Build history of the part. All positions in model axes, mm. A direction names the side the tool comes from. Round coordinates to 2 decimals unless told otherwise and drop trailing zeros. Write each loop counter-clockwise with the first axis right and the second up, starting at its lowest first coordinate (ties: lowest second). Pieces come first, ordered by that corner, then holes. Notation, with made-up numbers: M 23.25,38 L 72.25,38 A13 cw 72.25,61 Z; hole C 8.5,16 d2. An arc over 180 degrees is marked long. Use a Markdown table: item, result.
from build123d import *

# Parameters (mm, degrees)
F2_DEPTH    = 12.5
F3_T1_DEPTH = 46.550163213
F3_T3_DEPTH = 50.7168298797
F4_R        = 1
F4_R_2      = 0.99999


# Not quite as in the source:
# - a fillet or chamfer that OpenCascade refuses, or shapes differently, is made with other operations: its cross-section is extruded or revolved along the edge and cut away or added
# - a fillet or chamfer is up to 0.001 mm smaller than in the source, because OpenCascade refuses the exact size


with BuildPart() as f2:
    # F1 (on Front) → F2 (new body, symmetric)
    with BuildSketch(Plane.XZ):
        Polygon((0, 2), (0, 0), (20.8333333333, 0), (20.8333333333, 8), (18.3333333333, 8), (18.3333333333, 6), (15, 6), (15, 4), (10, 4), (10, 2), align=None)
    extrude(amount=F2_DEPTH, both=True)

    # F3: chamfer of 5 on 4 edges, made by hand

    # F3_s2 → F3_t1 (cut)
    with BuildSketch(Plane.YZ.offset(-12.8584149398)):
        Polygon((-12.5, 5), (-7.5, 0), (-12.5, 0), align=None)
        Polygon((7.5, 0), (12.5, 5), (12.5, 0), align=None)
    extrude(amount=F3_T1_DEPTH, mode=Mode.SUBTRACT)

    # F3_s4 → F3_t3 (cut)
    with BuildSketch(Plane.XZ.offset(-25.3584149398)):
        Polygon((0, 5), (5, 0), (0, 0), align=None)
        Polygon((20.8333333333, 5), (15.8333333333, 0), (20.8333333333, 0), align=None)
    extrude(amount=F3_T3_DEPTH, mode=Mode.SUBTRACT)

    # F4 (call 1 of 10: OpenCascade refuses the feature's edges together)
    f4_edges = [f2.edges().sort_by_distance(p)[0] for p in [
        (6.5, -9.5, 2),
    ]]
    fillet(f4_edges, radius=F4_R)

    # F4#2 (call 2 of 10)
    f4_2_edges = [f2.edges().sort_by_distance(p)[0] for p in [
        (12.5, -11.5, 4),
    ]]
    fillet(f4_2_edges, radius=F4_R)

    # F4#3 (call 3 of 10) (radius 1 in the source; OpenCascade refuses exactly that, so slightly less here)
    f4_3_edges = [f2.edges().sort_by_distance(p)[0] for p in [
        (16.666667, -12.5, 6),
    ]]
    fillet(f4_3_edges, radius=F4_R_2)

    # F4#4 (call 4 of 10)
    f4_4_edges = [f2.edges().sort_by_distance(p)[0] for p in [
        (19.583333, -12.5, 8),
    ]]
    fillet(f4_4_edges, radius=F4_R)

    # F4#5 (call 5 of 10)
    f4_5_edges = [f2.edges().sort_by_distance(p)[0] for p in [
        (19.583333, 12.5, 8),
    ]]
    fillet(f4_5_edges, radius=F4_R)

    # F4#6 (call 6 of 10) (radius 1 in the source; OpenCascade refuses exactly that, so slightly less here)
    f4_6_edges = [f2.edges().sort_by_distance(p)[0] for p in [
        (16.666667, 12.5, 6),
    ]]
    fillet(f4_6_edges, radius=F4_R_2)

    # F4#7 (call 7 of 10)
    f4_7_edges = [f2.edges().sort_by_distance(p)[0] for p in [
        (12.5, 11.5, 4),
    ]]
    fillet(f4_7_edges, radius=F4_R)

    # F4#8 (call 8 of 10)
    f4_8_edges = [f2.edges().sort_by_distance(p)[0] for p in [
        (6.5, 9.5, 2),
    ]]
    fillet(f4_8_edges, radius=F4_R)

    # F4#9 (call 9 of 10)
    f4_9_edges = [f2.edges().sort_by_distance(p)[0] for p in [
        (17.916667, -12.5, 5),
    ]]
    fillet(f4_9_edges, radius=F4_R)

    # F4#10 (call 10 of 10)
    f4_10_edges = [f2.edges().sort_by_distance(p)[0] for p in [
        (17.916667, 12.5, 5),
    ]]
    fillet(f4_10_edges, radius=F4_R)


solid = f2.part
Q1. Which spindle directions (+Z, -Z, +X, -X, +Y, -Y) get a long thin tool onto all of the face, cutting with end or side? Do faces 1 (the cylindrical face through (6.549, 8.003, 1.398)), 2 (the cylindrical face through (6.451, -8.003, 1.398)), 3 (the flat face through (17, 0, 6)), 4 (the flat face through (14.3, -9.3, 1.8)), 5 (the cylindrical face through (16.6, -12.1, 5.8)). Say none if no direction does.
Response values:
| item | result |
|---|---|
| face 1 | -X, +Y |
| face 2 | -X, -Y |
| face 3 | +Z, -X, +Y, -Y |
| face 4 | -Z, +X, -X, -Y |
| face 5 | +Z, -X, -Y |
Q2. Cut at A-A on y = -5.5. Give the cut face in (x, z).
Response values:
| item | result |
|---|---|
| outline | M 3,2 L 5,0 L 15.83,0 L 20.83,5 L 20.83,8 L 18.33,8 L 18.33,6 L 15,6 L 15,4 L 10,4 L 10,2 Z |
Q3. Drill centre lines: L1, parallel to X at y = -3.25, z = 5.75; L2, parallel to X at y = 5.5, z = 6.5; L3, parallel to Z at x = 13.5, y = -0.5. Where is each one in solid material? Low to high.
Response values:
| item | result |
|---|---|
| L1 | x = 15 to 20.83 |
| L2 | x = 18.33 to 20.83 |
| L3 | z = 0 to 4 |
Q4. Cut at B-B on x = 17.5. Give the cut face in (y, z).
Response values:
| item | result |
|---|---|
| outline | M -12.48,5.21 A1 ccw -12.21,4.71 L -9.17,1.67 L 9.17,1.67 L 12.21,4.71 A1 ccw 12.48,5.21 A1 ccw 11.5,6 L -11.5,6 A1 ccw Z |
Q5. Cut at D-D on x = 19.75. Give the cut face in (y, z).
Response values:
| item | result |
|---|---|
| outline | M -12.5,5.41 A1 ccw -12.21,4.71 L -11.42,3.92 L 11.42,3.92 L 12.21,4.71 A1 ccw 12.5,5.41 L 12.5,7 A1 ccw 11.5,8 L -11.5,8 A1 ccw -12.5,7 Z |
Q6. Drop flat-ended pins along their axis: P1, Ø7.5, axis at x = 6, y = -1, coming from the +Z side; P2, Ø3, axis at x = 13, y = 3.5, coming from the +Z side; P3, Ø4, axis at y = 4, z = 4.5, coming from the -X side. Give the stop position or say it passes through.
Response values:
| item | result |
|---|---|
| P1 | stops at z = 2 |
| P2 | stops at z = 4 |
| P3 | stops at x = 10 |
Q7. Cut at C-C on z = 2.75. Give the cut face in (x, y), and give its area (3 significant figures).
Response values:
| item | result |
|---|---|
| outline | M 10,-10.05 L 15,-10.05 L 15,-10.25 L 18.58,-10.25 L 18.58,10.25 L 15,10.25 L 15,10.05 L 10,10.05 Z |
| area | 174 mm2 |
